Autodesk Inventor part; units mm, degrees
ref_plane "YZ Plane" through (0, 0, 0) normal (1, 0, 0) x (0, 1, 0)
ref_plane "XZ Plane" through (0, 0, 0) normal (0, 1, 0) x (-1, 0, 0)
ref_plane "XY Plane" through (0, 0, 0) normal (0, 0, 1) x (1, 0, 0)
sketch "Sketch1" plane through (0, 0, 0) normal (0, 1, 0) x (-1, 0, 0)
  line L0 (0, 0) -> (19.05, 0)
  line L1 (19.05, 0) -> (19.05, -28.57)
  line L2 (19.05, -28.57) -> (0, -28.57)
  line L3 (0, -28.57) -> (0, 0)
  dimension "d0" = 19.05
  dimension "d1" = 28.57
extrude "Extrusion1" add sketch "Sketch1" along normal blind 3.43
sketch "Sketch2" plane through (0, 3.43, 0) normal (0, 1, 0) x (1, 0, 0)
  line L0 (0, 28.57) -> (-19.05, 28.57)
  line L1 (0, 0) -> (-9.53, 0)
  line L2 (-9.53, 0) -> (-9.53, 28.57)
  line L3 (-9.53, 28.57) -> (0, 28.57)
  line L4 (0, 28.57) -> (0, 0)
  dimension "d4" = 9.53
extrude "Extrusion2" add sketch "Sketch2" along normal blind 2.92
sketch "Sketch3" plane through (0, 6.35, 0) normal (0, 1, 0) x (1, 0, 0)
  line L0 (-15.75, 4.02) -> (-15.75, 8.66) construction
  line L1 (-14.16, 4.02) -> (-14.16, 8.66)
  line L2 (-17.34, 8.66) -> (-17.34, 4.02)
  arc A0 (-17.34, 4.02) -> (-14.16, 4.02) centre (-15.75, 4.02) ccw
  arc A1 (-14.16, 8.66) -> (-17.34, 8.66) centre (-15.75, 8.66) ccw
  line L3 (-19.05, 28.57) -> (-19.05, 0)
  line L4 (-15.75, 19.9) -> (-15.75, 24.54) construction
  line L5 (-14.16, 19.9) -> (-14.16, 24.54)
  line L6 (-17.34, 24.54) -> (-17.34, 19.9)
  arc A2 (-17.34, 19.9) -> (-14.16, 19.9) centre (-15.75, 19.9) ccw
  arc A3 (-14.16, 24.54) -> (-17.34, 24.54) centre (-15.75, 24.54) ccw
  line L7 (0, 28.57) -> (-9.53, 28.57)
  point P0 (0, 0)
  point P1 (-15.75, 6.34)
  point P2 (-15.75, 22.22)
  dimension "d7" = 4.64
  dimension "d8" = 3.18
  dimension "d9" = 3.3
  dimension "d10" = 4.64
  dimension "d11" = 3.18
  dimension "d12" = 15.88
  dimension "d13" = 6.35
  dimension "d16" = 3.3
extrude "Extrusion3" cut sketch "Sketch3" against normal through all
properties part number "59145_Actuator"
CAD build for the part. Positions are in the model's coordinates, mm. A direction names the side the tool comes from. Round coordinates to 2 decimals unless told otherwise and drop trailing zeros. Loops run counter-clockwise (first coordinate to the right, second up) from the corner with the lowest first, then second, coordinate; pieces in that order, holes last.
(1) Which spindle directions (+Z, -Z, +X, -X, +Y, -Y) get a long thin tool onto all of the face, cutting with end or side? Do faces 1 (the flat face through (-5, 6.35, -14)), 2 (the flat face through (-9.53, 5, -14)), 3 (the flat face through (-17.34, 2, -6)). Say none if no direction does.
(2) Wall check: line 1 along X through (y, z) = (3, -23); line 2 along Y through (x, z) = (-11.5, -7); line 3 along X through (y, z) = (6, -17.25). Give the ranges that are in metal, low to high.
(3) Drop flat-ended pins along their axis: pin 1 (1.5 mm diameter, centred on x = -16.5, y = 4.5, fed in from -Z); pin 2 (3 mm diameter, centred on x = -12, z = -7, fed in from +Y); pin 3 (1.5 mm diameter, centred on y = 5.5, z = -16.5, fed in from -X). Give the stop position or say it passes through.
(4) Cut at C-C (z = -18). Give the cut face in (x, y).
(5) Cut at D-D (z = -9.75). Give the cut face in (x, y).
(6) Cut at B-B (x = -15.75). Give the cut face in (y, z).
(7) Two-plate mould, pull along Z, no slides. Class faces 4 (the cylindrical face through (-15.72, 1.74, -10.25)), 5 (the flat face through (-14, 3.43, -14)), 6 (the flat face through (-8, 2, -28.57)): +Z half, -Z half, draft (parallel to the pull), parting line (faces both ways), or undercut.
(8) Cut at A-A (z = -24). Give the cut face in (x, y), plus the area to 3 significant figures.
Findings below:
1. face 1: +Z, -Z, +X, -X, +Y
1. face 2: +Z, -Z, -X, +Y
1. face 3: +Y, -Y
2. line 1: x = -19.05 to -17.34, -14.16 to 0
2. line 2: y = 0 to 3.43
2. line 3: x = -9.53 to 0
3. pin 1: passes through
3. pin 2: stops at y = 3.43
3. pin 3: stops at x = -9.53
4. outline: (-19.05, 0) - (0, 0) - (0, 6.35) - (-9.53, 6.35) - (-9.53, 3.43) - (-19.05, 3.43) - close
5. outline: (-19.05, 0) - (-16.91, 0) - (-16.91, 3.43) - (-19.05, 3.43) - close; (-14.59, 0) - (0, 0) - (0, 6.35) - (-9.53, 6.35) - (-9.53, 3.43) - (-14.59, 3.43) - close
6. outline: (0, -28.57) - (3.43, -28.57) - (3.43, -26.13) - (0, -26.13) - close; (0, -18.31) - (3.43, -18.31) - (3.43, -10.25) - (0, -10.25) - close; (0, -2.43) - (3.43, -2.43) - (3.43, 0) - (0, 0) - close
7. face 4: undercut
7. face 5: draft
7. face 6: -Z half
8. outline: (-19.05, 0) - (-17.34, 0) - (-17.34, 3.43) - (-19.05, 3.43) - close; (-14.16, 0) - (0, 0) - (0, 6.35) - (-9.53, 6.35) - (-9.53, 3.43) - (-14.16, 3.43) - close
8. area: 82.3 mm2
